from build123d import *

# Parameters (mm, degrees)
CUT_EXTRUDE1_START = -6.35
CUT_EXTRUDE1_DEPTH = 6.35


# Read off the part's stored shape, not the designer's step: Cut-Extrude1
with BuildPart() as part:
    # Sketch1 → Revolve1 (revolve)
    with BuildSketch(Plane(origin=(0, 0, 0), x_dir=(0, 0, -1), z_dir=(1, 0, 0)), mode=Mode.PRIVATE) as revolve1_sk:
        with BuildLine():
            Line((-3.175, 3.175), (3.175, 3.175))
            Line((3.175, 3.175), (3.175, 38.896804014))
            ThreePointArc((3.175, 38.896804014), (2.778125, 39.584211679), (1.984375, 39.584211679))
            ThreePointArc((1.984375, 39.584211679), (0, 39.0525), (-1.984375, 39.584211679))
            ThreePointArc((-1.984375, 39.584211679), (-2.778125, 39.584211679), (-3.175, 38.896804014))
            Line((-3.175, 38.896804014), (-3.175, 3.175))
        make_face()
    revolve(revolve1_sk.sketch.rotate(Axis((0, 0, -3.4925), (0, 0, 1)), 90), axis=Axis((0, 0, -3.4925), (0, 0, 1)))

    # Cut-Extrude1 outline → Cut-Extrude1 (cut)
    with BuildSketch(Plane.XY.offset(3.175).offset(CUT_EXTRUDE1_START)):
        with BuildLine():
            ThreePointArc((6.735192091, 6.735192091), (8.799952547, 3.645059693), (9.525, 0))
            add(Edge.make_bspline(
                [(9.525, 0), (9.525, 16.300780004), (-3.753785862, 16.300780004), (-3.753785862, 32.585930164), (6.859779029, 36.483664171), (17.706636116, 30.103665266)],
                knots=[0, 0, 0, 0, 0, 0, 1, 1, 1, 1, 1, 1], degree=5))
            ThreePointArc((17.706636116, 30.103665266), (-3.638359508, 34.734967469), (-23.560358803, 25.781100017))
            Line((-23.560358803, 25.781100017), (-23.560358803, 7.047534491))
            Line((-23.560358803, 7.047534491), (-8.568754556, 22.039138738))
            Line((-8.568754556, 22.039138738), (6.735192091, 6.735192091))
        make_face()
        with BuildLine():
            ThreePointArc((-6.735192091, 6.735192091), (-3.645059693, 8.799952547), (0, 9.525))
            add(Edge.make_bspline(
                [(0, 9.525), (-16.300780004, 9.525), (-16.300780004, -3.753785862), (-32.585930164, -3.753785862), (-36.483664171, 6.859779029), (-30.103665266, 17.706636116)],
                knots=[0, 0, 0, 0, 0, 0, 1, 1, 1, 1, 1, 1], degree=5))
            ThreePointArc((-30.103665266, 17.706636116), (-34.734967469, -3.638359508), (-25.781100017, -23.560358803))
            Line((-25.781100017, -23.560358803), (-7.047534491, -23.560358803))
            Line((-7.047534491, -23.560358803), (-22.039138738, -8.568754556))
            Line((-22.039138738, -8.568754556), (-6.735192091, 6.735192091))
        make_face()
        with BuildLine():
            ThreePointArc((6.735192091, -6.735192091), (3.645059693, -8.799952547), (0, -9.525))
            add(Edge.make_bspline(
                [(0, -9.525), (16.300780004, -9.525), (16.300780004, 3.753785862), (32.585930164, 3.753785862), (36.483664171, -6.859779029), (30.103665266, -17.706636116)],
                knots=[0, 0, 0, 0, 0, 0, 1, 1, 1, 1, 1, 1], degree=5))
            ThreePointArc((30.103665266, -17.706636116), (34.734967469, 3.638359508), (25.781100017, 23.560358803))
            Line((25.781100017, 23.560358803), (7.047534491, 23.560358803))
            Line((7.047534491, 23.560358803), (22.039138738, 8.568754556))
            Line((22.039138738, 8.568754556), (6.735192091, -6.735192091))
        make_face()
        with BuildLine():
            ThreePointArc((-6.735192091, -6.735192091), (-8.799952547, -3.645059693), (-9.525, 0))
            add(Edge.make_bspline(
                [(-9.525, 0), (-9.525, -16.300780004), (3.753785862, -16.300780004), (3.753785862, -32.585930164), (-6.859779029, -36.483664171), (-17.706636116, -30.103665266)],
                knots=[0, 0, 0, 0, 0, 0, 1, 1, 1, 1, 1, 1], degree=5))
            ThreePointArc((-17.706636116, -30.103665266), (3.638359508, -34.734967469), (23.560358803, -25.781100017))
            Line((23.560358803, -25.781100017), (23.560358803, -7.047534491))
            Line((23.560358803, -7.047534491), (8.568754556, -22.039138738))
            Line((8.568754556, -22.039138738), (-6.735192091, -6.735192091))
        make_face()
    extrude(amount=CUT_EXTRUDE1_DEPTH, mode=Mode.SUBTRACT)


solid = part.part
Here's how the part is built. I have some questions about the finished solid (model axes, mm). A direction names the side the tool comes from. Coordinates: 2 decimals unless noted, no trailing zeros.
Item 1: If we mould it in two halves opening along X, with no side actions, what happens to faces 3 (the cylindrical face through (8.78, 3.69, -0.04)), 4 (the flat face through (1, 8, 3.175))? For each: +X half, -X half, draft (parallel to the pull), parting line (faces both ways), or undercut.
Item 2: Will these pins go through, and if not, where does the flat tip stop? pin 1 (1.9 mm diameter, centred on x = 12.5, z = 0.5, fed in from -Y); pin 2 (1 mm diameter, centred on x = 14, z = 2, fed in from -Y); pin 3 (1.9 mm diameter, centred on y = -15, z = 0.5, fed in from -X).
Item 3: If I drill on line 1 (X direction, y = -20.5, z = 2.5); line 2 (X direction, y = 12, z = 0); line 3 (Y direction, x = -19, z = 0.25), over which ranges is the centre line in solid material (lowest first)?
Item 4: I want a section at A-A on z = 0.25. Count the separate pieces of the cut face and the enclosed holes in it, and give its area (3 significant figures).
Item 5: On a 3-axis mill with a long thin cutter (end or side, diameter ignored), from which of +Z, -Z, +X, -X, +Y, -Y can I reach the whole of each face in a straight line? I mean faces 1 (the flat face through (-1, 8, -3.175)), 2 (the flat face through (-1.02, 14.49, -0.04)). Say none if no direction works.
Findings below:
1. face 3: undercut
1. face 4: draft
2. pin 1: stops at y = -37.4
2. pin 2: stops at y = -37.29
2. pin 3: stops at x = -36.52
3. line 1: x = -33.98 to -28.28, -10.11 to -1.75, 7.03 to 10.11, 23.56 to 33.98
3. line 2: x = -37.16 to -32.8, -32.34 to -23.56, -18.61 to 1.47, 6.07 to 18.61, 32.8 to 37.16
3. line 3: y = -34.13 to -23.56, -11.61 to -5.53, 2.31 to 11.61, 29.3 to 34.13
4. separate pieces: 1
4. enclosed holes: 5
4. area: 2,820 mm2
5. face 1: -Z, +X, -X, +Y, -Y
5. face 2: +Z, -Z
